```python
from build123d import *

# Parameters (mm, degrees)
F0_W      = 203.2
F0_H      = 101.6
F1_DEPTH  = 101.6
F2_W      = 50.8
F2_H      = 50.8
F3_DEPTH  = 76.2
F4_W      = 50.8
F4_H      = 50.8
F5_DEPTH  = 76.2
F7_DEPTH  = 101.6
F9_DEPTH  = 101.6
F11_DEPTH = 101.6
F13_DEPTH = 101.6
F14_W     = 203.2
F14_H     = 50.8
F15_DEPTH = 50.8


with BuildPart() as f1:
    # F0 (on Front) → F1 (new body)
    with BuildSketch(Plane.XZ):
        with Locations((-3.634136, -9.485549)):
            Rectangle(F0_W, F0_H)
    extrude(amount=F1_DEPTH)

    # F2 (on face) → F3 (cut)
    with BuildSketch(Plane.XZ.offset(101.6)):
        with Locations((72.565864, -34.885549)):
            Rectangle(F2_W, F2_H)
    extrude(amount=-F3_DEPTH, mode=Mode.SUBTRACT)

    # F4 (on face) → F5 (cut)
    with BuildSketch(Plane.XZ.offset(101.6)):
        with Locations((-79.834136, -34.885549)):
            Rectangle(F4_W, F4_H)
    extrude(amount=-F5_DEPTH, mode=Mode.SUBTRACT)

    # F6 (on face) → F7 (cut)
    with BuildSketch(Plane.XZ.offset(101.6)):
        with BuildLine():
            Line((97.965864, 15.914451), (97.965864, 41.314451))
            Line((97.965864, 41.314451), (72.565864, 41.314451))
            ThreePointArc((72.565864, 41.314451), (90.526376, 33.874963), (97.965864, 15.914451))
        make_face()
    extrude(amount=-F7_DEPTH, mode=Mode.SUBTRACT)

    # F8 (on face) → F9 (cut)
    with BuildSketch(Plane.XZ.offset(101.6)):
        with BuildLine():
            Line((-79.834136, 41.314451), (-105.234136, 41.314451))
            Line((-105.234136, 41.314451), (-105.234136, 15.914451))
            ThreePointArc((-105.234136, 15.914451), (-97.794648, 33.874963), (-79.834136, 41.314451))
        make_face()
    extrude(amount=-F9_DEPTH, mode=Mode.SUBTRACT)

    # F10 (on face) → F11 (cut)
    with BuildSketch(Plane.XZ.offset(101.6)):
        with BuildLine():
            ThreePointArc((85.265864, 15.914451), (81.54612, 24.894707), (72.565864, 28.614451))
            ThreePointArc((72.565864, 28.614451), (63.585608, 6.934195), (85.265864, 15.914451))
        make_face()
    extrude(amount=-F11_DEPTH, mode=Mode.SUBTRACT)

    # F12 (on face) → F13 (cut)
    with BuildSketch(Plane.XZ.offset(101.6)):
        with BuildLine():
            ThreePointArc((-67.134136, 15.914451), (-70.85388, 24.894707), (-79.834136, 28.614451))
            ThreePointArc((-79.834136, 28.614451), (-88.814392, 6.934195), (-67.134136, 15.914451))
        make_face()
    extrude(amount=-F13_DEPTH, mode=Mode.SUBTRACT)

    # F14 (on face) → F15 (cut)
    with BuildSketch(Plane.XZ.offset(101.6)):
        with Locations((-3.634136, 15.914451)):
            Rectangle(F14_W, F14_H)
    extrude(amount=-F15_DEPTH, mode=Mode.SUBTRACT)


solid = f1.part
```
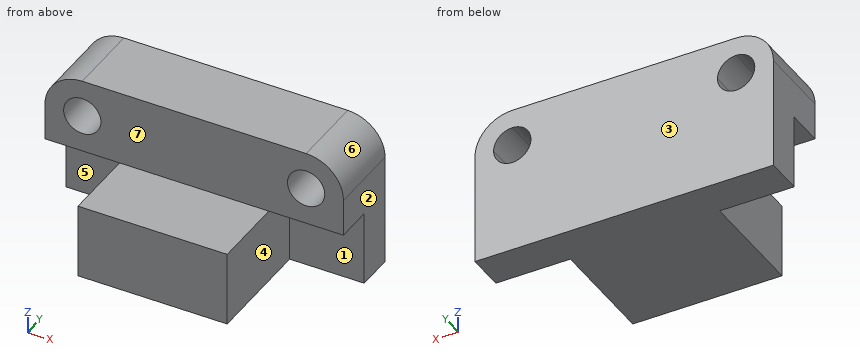
CAD build for the part. Positions are in the model's coordinates, mm. Face numbers are marked on the shaded views. A direction names the side the tool comes from. Give positions to 0.01 mm unless a question says otherwise; leave off trailing zeros. Loops run counter-clockwise (first coordinate to the right, second up) from the corner with the lowest first, then second, coordinate; pieces in that order, holes last. Notation, with made-up numbers: M 43,49 L 87,49 A23 ccw 87,71 Z; hole C 2.5,-40 d11. An arc over 180 degrees is marked long. Use one line per item in the form item = value.
Item 1: Flat gauge pins, fed straight in: pin 1 (3 mm diameter, centred on x = 33.5, z = 5.5, fed in from -Y); pin 2 (2 mm diameter, centred on x = -29, z = -18, fed in from +Y); pin 3 (3 mm diameter, centred on y = -39, z = -27.5, fed in from -X); pin 4 (7.5 mm diameter, centred on x = -92.5, y = -44, fed in from -Z). Where does each tip first touch, or does it go through?
Determined:
pin_1 = -50.8
pin_2 = 0
pin_3 = -54.43
pin_4 = -9.49
Item 2: Slice it at B-B (z = -44.5). List the corners of the cut face in (x, y).
Determined:
outline = M -105.23,-25.4 L -54.43,-25.4 L -54.43,-101.6 L 47.17,-101.6 L 47.17,-25.4 L 97.97,-25.4 L 97.97,0 L -105.23,0 Z
Item 3: Two-plate mould, pull along Y, no slides. Class the marked faces 1, 2 and 3: pulls with the +Y half, pulls with the -Y half, needs draft (parallel to the pull), parting line crosses it, or undercut.
Determined:
face_1 = pulls with the -Y half
face_2 = needs draft
face_3 = pulls with the +Y half
Item 4: Slice it at A-A (y = -45.5). List the corners of the cut face in (x, z), plus the area to 3 significant figures.
Determined:
outline = M -105.23,-9.49 L -54.43,-9.49 L -54.43,-60.29 L 47.17,-60.29 L 47.17,-9.49 L 97.97,-9.49 L 97.97,15.91 A25.4 ccw 72.57,41.31 L -79.83,41.31 A25.4 ccw -105.23,15.91 Z; hole C -79.83,15.91 d25.4; hole C 72.57,15.91 d25.4
area = 14,200 mm2
Item 5: Drill centre lines: probe 1 along Y at (x, z) = (-75.5, -34.5); probe 2 along Y at (x, z) = (-64, 11); probe 3 along Z at (x, y) = (81, -9.5). Where is each one in solid material? Low to high. Write a range as from..to.
Determined:
probe_1 = -25.4..0
probe_2 = -50.8..0
probe_3 = -60.29..6.42, 25.41..39.87
Item 6: Slice it at C-C (z = 25). List the corners of the cut face in (x, y), plus the area to 3 significant figures.
Determined:
outline = M -103.55,-50.8 L -88.71,-50.8 L -88.71,0 L -103.55,0 Z; M -70.96,-50.8 L 63.69,-50.8 L 63.69,0 L -70.96,0 Z; M 81.44,-50.8 L 96.29,-50.8 L 96.29,0 L 81.44,0 Z
area = 8,350 mm2
Item 7: Slice it at D-D (x = 51). List the corners of the cut face in (y, z).
Determined:
outline = M -50.8,-9.49 L -25.4,-9.49 L -25.4,-60.29 L 0,-60.29 L 0,41.31 L -50.8,41.31 Z
Item 8: Which spindle directions (+Z, -Z, +X, -X, +Y, -Y) get a long thin tool onto all of the face, cutting with end or side? Do the marked faces 4, 5, 6 and 7. Say none if no direction does.
Determined:
face_4 = -Z, +X, -Y
face_5 = -Z, -X, -Y
face_6 = +Z, +X, +Y, -Y
face_7 = +Z, +X, -X, -Y
